Here's how the part is built. I have some questions about the finished solid (model axes, mm). Face numbers are marked on the shaded views. A direction names the side the tool comes from. Round coordinates to 2 decimals unless told otherwise and drop trailing zeros. Write each loop counter-clockwise with the first axis right and the second up, starting at its lowest first coordinate (ties: lowest second). Pieces come first, ordered by that corner, then holes. Notation, with made-up numbers: (4, -18.75) -> (46, -18.75) arc R24 cw to (46, 18.25) -> close; hole circle Ø8 at (5, 5). An arc over 180 degrees is marked (long way). Answer in a Markdown table with one row per item.
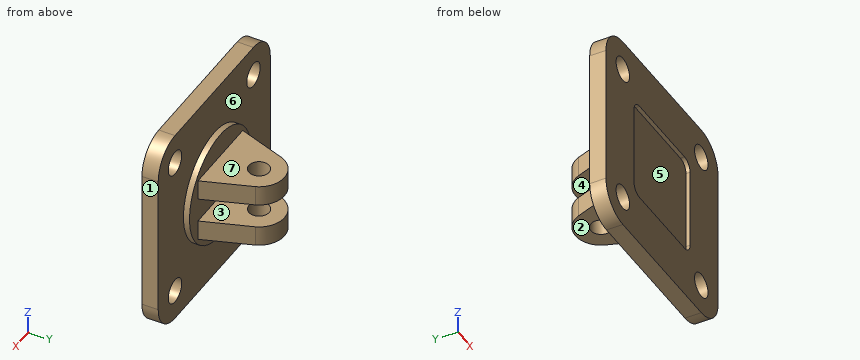
from build123d import *

# Parameters (mm, degrees)
EXTRUDE_3_DEPTH             = 8
SKETCH_4_R                  = 27.5
EXTRUDE_4_DEPTH             = 3
SKETCH_6_R                  = 6
CUT_EXTRUDE_1_DEPTH         = 72.161787499
PATTERN_LINEAR_1_COUNT      = 2
PATTERN_LINEAR_1_PITCH      = 70
PATTERN_LINEAR_1_COUNT_DIR2 = 2
PATTERN_LINEAR_1_PITCH_DIR2 = 70
CUT_EXTRUDE_2_DEPTH         = 2
SKETCH_13_R                 = 5
EXTRUDE_6_DEPTH             = 16
SKETCH_14_W                 = 40
SKETCH_14_H                 = 35
CUT_EXTRUDE_3_DEPTH         = 6


with BuildPart() as part:
    # 草圖3 → 填料-伸長3 (new body)
    with BuildSketch(Plane(origin=(0, 0, 0), x_dir=(1, 0, 0), z_dir=(0, 1, 0))):
        with BuildLine():
            Line((35, 50), (-35, 50))
            ThreePointArc((-35, 50), (-45.606601718, 45.606601718), (-50, 35))
            Line((-50, 35), (-50, -35))
            ThreePointArc((-50, -35), (-45.606601718, -45.606601718), (-35, -50))
            Line((-35, -50), (35, -50))
            ThreePointArc((35, -50), (45.606601718, -45.606601718), (50, -35))
            Line((50, -35), (50, 35))
            ThreePointArc((50, 35), (45.606601718, 45.606601718), (35, 50))
        make_face()
    extrude(amount=EXTRUDE_3_DEPTH)

    # 草圖4 → 填料-伸長4 (add)
    with BuildSketch(Plane(origin=(0, 8, 0), x_dir=(1, 0, 0), z_dir=(0, 1, 0))):
        with Locations(Location((0, 0, 0), (0, 0, 270))):
            Circle(SKETCH_4_R)
    extrude(amount=EXTRUDE_4_DEPTH)

    # 草圖6 → 除料-伸長1 (cut, through all)
    with BuildSketch(Plane(origin=(0, 8, 0), x_dir=(1, 0, 0), z_dir=(0, 1, 0))):
        with Locations(Location((-35, 35, 0), (0, 0, 270))):
            Circle(SKETCH_6_R)
    cut_extrude_1 = extrude(amount=-CUT_EXTRUDE_1_DEPTH, mode=Mode.SUBTRACT)

    # 直線複製排列1: Cut-Extrude 1 2 × 2
    with Locations(*[(i * PATTERN_LINEAR_1_PITCH, 0, j * PATTERN_LINEAR_1_PITCH_DIR2) for i in range(PATTERN_LINEAR_1_COUNT) for j in range(PATTERN_LINEAR_1_COUNT_DIR2) if (i, j) != (0, 0)]):
        add(cut_extrude_1, mode=Mode.SUBTRACT)

    # 草圖9 → 除料-伸長2 (cut)
    with BuildSketch(Plane.XZ):
        with BuildLine():
            Line((-20, -25), (20, -25))
            ThreePointArc((20, -25), (23.535533906, -23.535533906), (25, -20))
            Line((25, -20), (25, 20))
            ThreePointArc((25, 20), (23.535533906, 23.535533906), (20, 25))
            Line((20, 25), (-20, 25))
            ThreePointArc((-20, 25), (-23.535533906, 23.535533906), (-25, 20))
            Line((-25, 20), (-25, -20))
            ThreePointArc((-25, -20), (-23.535533906, -23.535533906), (-20, -25))
        make_face()
    extrude(amount=-CUT_EXTRUDE_2_DEPTH, mode=Mode.SUBTRACT)

    # 草圖13 → 填料-伸長6 (add, symmetric)
    with BuildSketch(Plane.XY):
        with BuildLine():
            Line((-20, 11), (20, 11))
            Line((20, 11), (11.638479247, 34.560241312))
            ThreePointArc((11.638479247, 34.560241312), (0, 42.5), (-11.638479247, 34.560241312))
            Line((-11.638479247, 34.560241312), (-20, 11))
        make_face()
        with Locations((0, 30)):
            Circle(SKETCH_13_R, mode=Mode.SUBTRACT)
    extrude(amount=EXTRUDE_6_DEPTH, both=True)

    # 草圖14 → 除料-伸長3 (cut, symmetric)
    with BuildSketch(Plane.XY):
        with Locations((0, 28.5)):
            Rectangle(SKETCH_14_W, SKETCH_14_H)
    extrude(amount=CUT_EXTRUDE_3_DEPTH, both=True, mode=Mode.SUBTRACT)


solid = part.part
1) I want a section at A-A, the plane y = 6. List the corners of the cut face in (x, z) for me.
Response:
| item | result |
|---|---|
| outline | (-50, -35) arc R15 ccw to (-35, -50) -> (35, -50) arc R15 ccw to (50, -35) -> (50, 35) arc R15 ccw to (35, 50) -> (-35, 50) arc R15 ccw to (-50, 35) -> close; hole circle Ø12 at (-35, -35); hole circle Ø12 at (-35, 35); hole circle Ø12 at (35, -35); hole circle Ø12 at (35, 35) |
2) I need wall thicknesses on line 1 (X direction, y = 2.75, z = -35); line 2 (Z direction, x = 5, y = 12); line 3 (Y direction, x = 42, z = 8.5). Which ranges of each line are inside material? Lowest first, please. Write a range as [from, to].
Response:
| item | result |
|---|---|
| line 1 | x = [-50, -41], [-29, 29], [41, 50] |
| line 2 | z = [-16, -6], [6, 16] |
| line 3 | y = [0, 8] |
3) We'd pull the mould along Z, two halves only. Please class the marked faces 1, 2 and 3: +Z half, -Z half, draft (parallel to the pull), parting line (faces both ways), or undercut.
Response:
| item | result |
|---|---|
| face 1 | draft |
| face 2 | -Z half |
| face 3 | undercut |
4) Which directions (+Z, -Z, +X, -X, +Y, -Y) give clear straight access to the entire face, cutting with the end or side of a thin tool? Please do the marked faces 4, 5, 6 and 7.
Response:
| item | result |
|---|---|
| face 4 | +X, -X, +Y |
| face 5 | -Y |
| face 6 | +Y |
| face 7 | +Z, +X, -X, +Y |
5) I want a section at C-C, the plane y = 30. List the corners of the cut face in (x, z) for me.
Response:
| item | result |
|---|---|
| outline | (-13.26, -16) -> (-5, -16) -> (-5, -6) -> (-13.26, -6) -> close; (-13.26, 6) -> (-5, 6) -> (-5, 16) -> (-13.26, 16) -> close; (5, -16) -> (13.26, -16) -> (13.26, -6) -> (5, -6) -> close; (5, 6) -> (13.26, 6) -> (13.26, 16) -> (5, 16) -> close |
6) For pin 1 (13 mm diameter, centred on x = 0, y = 30, fed in from +Z); pin 2 (4 mm diameter, centred on x = 33.5, z = -7, fed in from +Y); pin 3 (7 mm diameter, centred on x = -35, z = -35, fed in from -Y); pin 4 (9.5 mm diameter, centred on x = 0.5, y = 21.5, fed in from -Z), each with a flat end and sliding along its axis, tell me the tip position at first contact or that it passes through.
Response:
| item | result |
|---|---|
| pin 1 | stops at z = 16 |
| pin 2 | stops at y = 8 |
| pin 3 | passes through |
| pin 4 | stops at z = -16 |
7) I want a section at D-D, the plane z = 0. List the corners of the cut face in (x, y) for me, and give its area (3 significant figures).
Response:
| item | result |
|---|---|
| outline | (-50, 0) -> (-25, 0) -> (-25, 2) -> (25, 2) -> (25, 0) -> (50, 0) -> (50, 8) -> (27.5, 8) -> (27.5, 11) -> (-27.5, 11) -> (-27.5, 8) -> (-50, 8) -> close |
| area | 865 mm^2 |
8) I want a section at B-B, the plane z = 31.5. List the corners of the cut face in (x, y) for me.
Response:
| item | result |
|---|---|
| outline | (-50, 0) -> (-39.87, 0) -> (-39.87, 8) -> (-50, 8) -> close; (-30.13, 0) -> (30.13, 0) -> (30.13, 8) -> (-30.13, 8) -> close; (39.87, 0) -> (50, 0) -> (50, 8) -> (39.87, 8) -> close |
